```python
from build123d import *

# Parameters (mm, degrees)
F_0_1MM_FIT_FOR_POT_R   = 10.5
BOSS_EXTRUDE1_DEPTH     = 2.75
SKETCH4_R               = 10.5
SKETCH4_R_2             = 8.275
BOSS_EXTRUDE2_DEPTH     = 4.25
BOSS_EXTRUDE3_DEPTH     = 2
FILLET1_R               = 0.25
BOSS_EXTRUDE6_DEPTH     = 10
BOSS_EXTRUDE7_DEPTH     = 2.9
BOSS_EXTRUDE8_DEPTH     = 3
FILLET2_R               = 1.5
BOSS_EXTRUDE9_DEPTH     = 17.5
SKETCH11_W              = 12.5
SKETCH11_H              = 6
CUT_EXTRUDE1_DEPTH      = 81.518110176
CUT_EXTRUDE1_DEPTH_BACK = 81.518110176


with BuildPart() as part:
    # 0.1mm fit for pot → Boss-Extrude1 (new body)
    with BuildSketch(Plane(origin=(0, 0, 0), x_dir=(1, 0, 0), z_dir=(0, 1, 0))):
        with Locations(Location((0, 0, 0), (0, 0, 270))):
            Circle(F_0_1MM_FIT_FOR_POT_R)
    extrude(amount=BOSS_EXTRUDE1_DEPTH)

    # Sketch4 → Boss-Extrude2 (add)
    with BuildSketch(Plane(origin=(0, 2.75, 0), x_dir=(1, 0, 0), z_dir=(0, 1, 0))):
        with Locations(Location((0, 0, 0), (0, 0, 270))):
            Circle(SKETCH4_R)
        with Locations(Location((0, 0, 0), (0, 0, 270))):
            Circle(SKETCH4_R_2, mode=Mode.SUBTRACT)
    extrude(amount=BOSS_EXTRUDE2_DEPTH)

    # Sketch5 → Boss-Extrude3 (add)
    with BuildSketch(Plane(origin=(0, 2.75, 0), x_dir=(1, 0, 0), z_dir=(0, 1, 0))):
        with BuildLine():
            Line((-1, -8.214354813), (-1, -7.065799598))
            Line((-1, -7.065799598), (0.988059701, -7.065799598))
            Line((0.988059701, -7.065799598), (0.988059701, -8.215799598))
            ThreePointArc((0.988059701, -8.215799598), (-0.006013695, -8.274997815), (-1, -8.214354813))
        make_face()
    extrude(amount=BOSS_EXTRUDE3_DEPTH)

    # Fillet1
    fillet1_edges = [part.edges().sort_by_distance(p)[0] for p in [
        (0.988059701, 3.75, 7.065799598),
        (-1, 3.75, 7.065799598),
        (-0.005970149, 4.75, 7.065799598),
        (-1, 4.75, 7.640077205),
        (0.988059701, 4.75, 7.640799598),
    ]]
    fillet(fillet1_edges, radius=FILLET1_R)

    # Sketch7 → Boss-Extrude6 (add)
    with BuildSketch(Plane(origin=(0, 7, 0), x_dir=(1, 0, 0), z_dir=(0, 1, 0))):
        with BuildLine():
            Line((3.299602194, 9.968080325), (3.299602194, 8.373328213))
            ThreePointArc((3.299602194, 8.373328213), (-9, 0), (3.299602194, -8.373328213))
            Line((3.299602194, -8.373328213), (3.299602194, -9.968080325))
            ThreePointArc((3.299602194, -9.968080325), (-10.5, 0), (3.299602194, 9.968080325))
        make_face()
    extrude(amount=BOSS_EXTRUDE6_DEPTH)

    # Sketch8 → Boss-Extrude7 (add)
    with BuildSketch(Plane(origin=(0, 17, 0), x_dir=(1, 0, 0), z_dir=(0, 1, 0))):
        with BuildLine():
            Line((3.299602194, 12.315645552), (3.299602194, 9.968080325))
            ThreePointArc((3.299602194, 9.968080325), (-10.5, 0), (3.299602194, -9.968080325))
            Line((3.299602194, -9.968080325), (3.299602194, -12.315645552))
            ThreePointArc((3.299602194, -12.315645552), (-12.75, 0), (3.299602194, 12.315645552))
        make_face()
    extrude(amount=-BOSS_EXTRUDE7_DEPTH)

    # Sketch9 → Boss-Extrude8 (add)
    with BuildSketch(Plane.XZ):
        with BuildLine():
            Line((-9.3641604, 4.75), (-59.3641604, 4.75))
            Line((-59.3641604, 4.75), (-59.3641604, -4.75))
            Line((-59.3641604, -4.75), (-9.3641604, -4.75))
            ThreePointArc((-9.3641604, -4.75), (-10.5, 0), (-9.3641604, 4.75))
        make_face()
    extrude(amount=-BOSS_EXTRUDE8_DEPTH)

    # Fillet2
    fillet2_edges = [part.edges().sort_by_distance(p)[0] for p in [
        (-10.5, 3, 0),
        (-9.3641604, 1.5, 4.75),
        (-9.3641604, 1.5, -4.75),
    ]]
    fillet(fillet2_edges, radius=FILLET2_R)

    # Sketch10 → Boss-Extrude9 (add)
    with BuildSketch(Plane.ZY.offset(59.3641604)):
        with BuildLine():
            Line((-45, -22), (-43, -22))
            add(Edge.make_bspline(
                [(-4.75, 0), (-26.762186457, -1.948698647), (-43, -22)],
                knots=[0.548592822, 0.548592822, 0.548592822, 1, 1, 1], degree=2))
            Line((-4.75, 0), (4.75, 0))
            add(Edge.make_bspline(
                [(43, -22), (26.762186461, -1.948698647), (4.75, 0)],
                knots=[0, 0, 0, 0.451407178, 0.451407178, 0.451407178], degree=2))
            Line((43, -22), (45, -22))
            add(Edge.make_bspline(
                [(4.75, 3), (28.386779804, 0.912348176), (45, -22)],
                knots=[0.545557352, 0.545557352, 0.545557352, 1, 1, 1], degree=2))
            Line((4.75, 3), (-4.75, 3))
            add(Edge.make_bspline(
                [(-45, -22), (-28.386779803, 0.912348176), (-4.75, 3)],
                knots=[0, 0, 0, 0.454442648, 0.454442648, 0.454442648], degree=2))
        make_face()
    extrude(amount=-BOSS_EXTRUDE9_DEPTH)

    # Sketch11 → Cut-Extrude1 (cut, two sides)
    with BuildSketch(Plane(origin=(0, 0, -4.75), x_dir=(-1, 0, 0), z_dir=(0, 0, -1))) as cut_extrude1_sk:
        with Locations((50.6141604, -17)):
            Rectangle(SKETCH11_W, SKETCH11_H)
    extrude(amount=CUT_EXTRUDE1_DEPTH, mode=Mode.SUBTRACT)
    extrude(cut_extrude1_sk.sketch, amount=-CUT_EXTRUDE1_DEPTH_BACK, mode=Mode.SUBTRACT)


solid = part.part
```
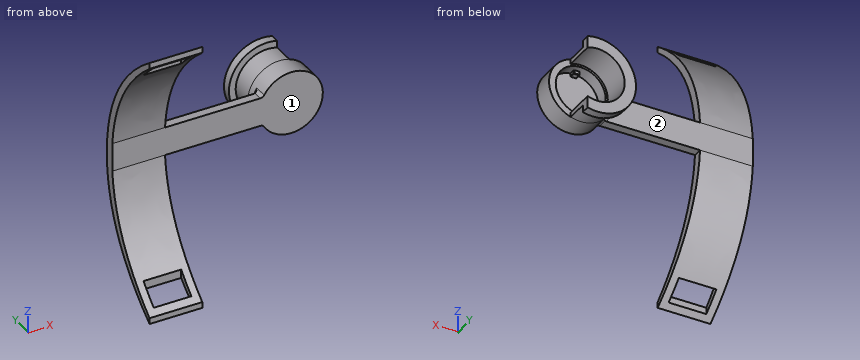
Check sheet for the modelled part. Datum: model origin and axes. Units: mm. Face numbers are marked on the shaded views. Round coordinates to 2 decimals unless told otherwise and drop trailing zeros. Loops run counter-clockwise (first coordinate to the right, second up) from the corner with the lowest first, then second, coordinate; pieces in that order, holes last. Notation, with made-up numbers: M 43.5,76.5 L 64.5,76.5 A25 cw 64.5,93.5 Z; hole C -38.75,4 d1. An arc over 180 degrees is marked long. Answer as a JSON object with one key per item and string values.
1. Section check D-D (x = -3.5). Record the boundary of the cut face in (y, z).
Reply:
{"outline": "M 0,-9.9 L 14.1,-9.9 L 14.1,-12.26 L 17,-12.26 L 17,-8.29 L 7,-8.29 L 7,-7.5 L 2.75,-7.5 L 2.75,7.5 L 7,7.5 L 7,8.29 L 17,8.29 L 17,12.26 L 14.1,12.26 L 14.1,9.9 L 0,9.9 Z"}
2. Section check A-A (z = 0). Record the boundary of the cut face in (x, y) (3 decimals), plus the area to 3 significant figures.
Reply:
{"outline": "M -59.364,0 L 10.5,0 L 10.5,7 L 8.275,7 L 8.275,2.75 L -8.275,2.75 L -8.275,7 L -9,7 L -9,17 L -12.75,17 L -12.75,14.1 L -10.5,14.1 L -10.5,4.5 A1.5 cw -12,3 L -59.364,3 Z", "area": "245 mm²"}
3. Gauge pin test, flat ends, axial feed: P1, Ø8, axis at x = -44.5, z = 4.5, coming from the -Y side; P2, Ø6.5, axis at y = -17, z = -40.5, coming from the +X side; P3, Ø8, axis at x = -44, z = -26, coming from the +Y side. Record the tip position at first contact, or that the pin passes through.
Reply:
{"P1": "stops at y = -0.47", "P2": "stops at x = -41.86", "P3": "stops at y = -1.74"}
4. Section check C-C (y = 9). Record the boundary of the cut face in (x, z), plus the area to 3 significant figures.
Reply:
{"outline": "M 3.3,-9.97 L 3.3,-8.37 A9 cw long 3.3,8.37 L 3.3,9.97 A10.5 ccw long Z", "area": "56.0 mm²"}
5. Scan lines: line 1 (X direction, y = 5.05, z = 0) (3 decimals); line 2 (Z direction, x = 0, y = 11); line 3 (Y direction, x = 3, z = 9). Record each from-to range of solid material in increasing order.
Reply:
{"line 1": "x = -10.5 to -8.275, 8.275 to 10.5", "line 2": "z = -10.5 to -9, 9 to 10.5", "line 3": "y = 0 to 17"}
6. Mould release check, pull along Z, two halves, no side actions. Record for the marked faces 1 and 2: pulls with the +Z half, pulls with the -Z half, needs draft (parallel to the pull), parting line crosses it, or undercut.
Reply:
{"face 1": "undercut", "face 2": "needs draft"}
7. Section check B-B (x = -52). State how many separate pieces and enclosed holes the cut face has, plus the area to 3 significant figures.
Reply:
{"separate pieces": "3", "enclosed holes": "0", "area": "228 mm²"}
